from build123d import *

# Parameters (mm, degrees)
PAD_DEPTH       = 17
PAD001_DEPTH    = 2
PAD002_DEPTH    = 1.8
SKETCH003_W     = 32
SKETCH003_H     = 8
PAD003_DEPTH    = 5
SKETCH004_W     = 3.25
SKETCH004_H     = 3.25
POCKET_DEPTH    = 3.1
SKETCH005_W     = 6.497684
SKETCH005_H     = 9.461539
SKETCH005_W_2   = 6.809606
SKETCH005_H_2   = 19.151065
PAD004_DEPTH    = 0.225
CHAMFER_SIZE    = 4
SKETCH006_R     = 0.375
PAD005_DEPTH    = 16
POCKET001_DEPTH = 3
POCKET002_DEPTH = 3
SKETCH009_W     = 42
SKETCH009_H     = 2
PAD006_DEPTH    = 3
CHAMFER001_SIZE = 2


with BuildPart() as part:
    # Sketch → Pad (new body)
    with BuildSketch(Plane.XY):
        with BuildLine():
            Line((-10, 0), (-10, 5))
            Line((-10, 5), (5, 5))
            Line((5, 5), (5, -10))
            Line((5, -10), (0, -10))
            Line((0, -7.05), (0, -10))
            Line((0, -7.05), (0.143534, -7.05))
            ThreePointArc((0.143534, -7.05), (3.05, -6.3), (0.143534, -5.55))
            Line((0, -5.55), (0.143534, -5.55))
            Line((0, 0), (0, -5.55))
            Line((0, 0), (-5.55, 0))
            Line((-5.55, 0), (-5.55, 0.143534))
            ThreePointArc((-5.55, 0.143534), (-6.3, 3.05), (-7.05, 0.143534))
            Line((-7.05, 0), (-7.05, 0.143534))
            Line((-10, 0), (-7.05, 0))
        make_face()
    extrude(amount=-PAD_DEPTH)

    # Sketch001 (on Face16 of Pad) → Pad001 (join)
    with BuildSketch(Plane(origin=(0, 0, -17), x_dir=(1, 0, 0), z_dir=(0, 0, -1))):
        Polygon((5, -5), (-10, -5), (-10, 0), (0, 10), (5, 10), align=None)
    extrude(amount=PAD001_DEPTH)

    # Sketch002 (on Face1 of Pad001) → Pad002 (join)
    with BuildSketch(Plane.XY):
        Polygon((0, -10), (0, 0), (-10, 0), align=None)
    extrude(amount=-PAD002_DEPTH)

    # Sketch003 (on Face10 of Pad002) → Pad003 (join)
    with BuildSketch(Plane.XZ):
        with Locations((-26, -15)):
            Rectangle(SKETCH003_W, SKETCH003_H)
    extrude(amount=-PAD003_DEPTH)

    # Sketch004 (on Face22 of Pad003) → Pocket (cut)
    with BuildSketch(Plane.XZ):
        with Locations((-37.375, -13.375)):
            Rectangle(SKETCH004_W, SKETCH004_H)
    extrude(amount=-POCKET_DEPTH, mode=Mode.SUBTRACT)

    # Sketch005 → Pad004 (join)
    with BuildSketch(Plane(origin=(0, 0, -19), x_dir=(1, 0, 0), z_dir=(0, 0, -1))):
        with Locations((-40.563391, -2.425933)):
            Rectangle(SKETCH005_W, SKETCH005_H)
        with Locations((3.404803, 2.422745)):
            Rectangle(SKETCH005_W_2, SKETCH005_H_2)
    extrude(amount=-PAD004_DEPTH)

    # Chamfer
    chamfer_edges = [part.edges().sort_by_distance(p)[0] for p in [
        (-10, 2.5, -11),
        (5, 5, -9.3875),
    ]]
    chamfer(chamfer_edges, length=CHAMFER_SIZE)

    # Sketch006 (on Face29 of Chamfer) → Pad005 (join)
    with BuildSketch(Plane.XY.offset(-17)):
        with Locations((-6, -3)):
            Circle(SKETCH006_R)
        with Locations((-3, -6)):
            Circle(SKETCH006_R)
    extrude(amount=PAD005_DEPTH)

    # Sketch007 (on Face2 of Pad005) → Pocket001 (cut, symmetric)
    with BuildSketch(Plane.YZ.offset(5)):
        with BuildLine():
            ThreePointArc((-5.25, -5), (-6.25, -4), (-7.25, -5))
            Line((-7.25, -5), (-7.25, -14))
            ThreePointArc((-7.25, -14), (-6.25, -15), (-5.25, -14))
            Line((-5.25, -5), (-5.25, -14))
        make_face()
    extrude(amount=POCKET001_DEPTH, both=True, mode=Mode.SUBTRACT)

    # Sketch008 (on Face5 of Pocket001) → Pocket002 (cut)
    with BuildSketch(Plane(origin=(0, 5, 0), x_dir=(-1, 0, 0), z_dir=(0, 1, 0))):
        with BuildLine():
            ThreePointArc((7.25, -5), (6.25, -4), (5.25, -5))
            Line((5.25, -5), (5.25, -14))
            ThreePointArc((5.25, -14), (6.25, -15), (7.25, -14))
            Line((7.25, -5), (7.25, -14))
        make_face()
    extrude(amount=-POCKET002_DEPTH, mode=Mode.SUBTRACT)

    # Sketch009 (on Face35 of Pocket002) → Pad006 (join)
    with BuildSketch(Plane.XZ):
        with Locations((-21, -18)):
            Rectangle(SKETCH009_W, SKETCH009_H)
    extrude(amount=PAD006_DEPTH)

    # Chamfer001
    chamfer001_edges = [part.edges().sort_by_distance(p)[0] for p in [
        (-42, -3, -18),
    ]]
    chamfer(chamfer001_edges, length=CHAMFER001_SIZE)


solid = part.part
Input: part model. Units: mm. Frame: model coordinates. A direction names the side the tool comes from. Coordinates: 2 decimals unless noted, no trailing zeros. Order: outer loops, then holes, each group sorted by start corner. A loop starts at its lowest first (then second) coordinate and runs counter-clockwise, first axis right, second up.
1. Cut plane D-D, the plane x = 1.5. Return loops of the section in (y, z) (3 decimals), plus the area to 3 significant figures.
Checked values:
outline: (-11.998, -19) - (7.153, -19) - (7.153, -18.775) - (4.5, -18.775) - (4.5, 0) - (-4.75, 0) - (-4.75, -17) - (-7.85, -17) - (-7.85, 0) - (-10, 0) - (-10, -18.775) - (-11.998, -18.775) - close
area: 224 mm2
2. Cut plane C-C, the plane x = -16. Return loops of the section in (y, z), plus the area to 3 significant figures.
Checked values:
outline: (-3, -19) - (5, -19) - (5, -11) - (0, -11) - (0, -17) - (-3, -17) - close
area: 46.0 mm2
3. Access query for faces 4 (the flat face through (-24, -3, -18)), 5 (the cylindrical face through (3.8, -6.3, -15)), 6 (the flat face through (0, -3, -9)). Directions: +Z, -Z, +X, -X, +Y, -Y. A direction counts if a zero-diameter tool reaches every point of the face in a straight line with its end or side. Return the directions, or none.
Checked values:
face 4: +Z, -Z, -X, -Y
face 5: +X
face 6: -Y
4. Cut plane B-B, the plane z = -3.25. Return loops of the section in (x, y) (3 decimals).
Checked values:
outline: (-10, 0) - (-7.05, 0) - (-7.05, 0.144) arc R1.55 cw (long way) to (-5.55, 0.144) - (-5.55, 0) - (0, 0) - (0, -5.55) - (0.144, -5.55) arc R1.55 cw (long way) to (0.144, -7.05) - (0, -7.05) - (0, -10) - (5, -10) - (5, 1) - (1, 5) - (-10, 5) - close; circle Ø0.75 at (-6, -3); circle Ø0.75 at (-3, -6)
5. Cut plane A-A, the plane z = -9.25. Return loops of the section in (x, y) (3 decimals), plus the area to 3 significant figures.
Checked values:
outline: (-12.25, 0) - (-7.05, 0) - (-7.05, 0.144) arc R1.55 cw to (-7.25, 2.725) - (-7.25, 5) - (-12.25, 5) - close; circle Ø0.75 at (-6, -3); (-5.55, 0) - (0, 0) - (0, -5.55) - (0.144, -5.55) arc R1.55 cw to (2.64, -5.25) - (5, -5.25) - (5, 1) - (1, 5) - (-5.25, 5) - (-5.25, 2.64) arc R1.55 cw to (-5.55, 0.144) - close; circle Ø0.75 at (-3, -6); (0, -10) - (5, -10) - (5, -7.25) - (2.725, -7.25) arc R1.55 cw to (0.144, -7.05) - (0, -7.05) - close
area: 106 mm2
6. Draft query along Y for faces 1 (the flat face through (2, -10, -9)), 2 (the flat face through (-1, -1, 0)), 3 (the cylindrical face through (3.8, -6.2, -4)). Return one class per face: +Y half, -Y half, draft (parallel to the pull), parting line (faces both ways), or undercut.
Checked values:
face 1: -Y half
face 2: draft
face 3: undercut
7. Contact query for flat-ended pins moving along their axis: P1, Ø2.5, axis at x = 3.5, z = -10.5, coming from the -Y side; P2, Ø0.6, axis at x = -16, z = -18, coming from the -Y side; P3, Ø6, axis at x = -16, y = -5, coming from the +Z side. Output: stop coordinate, or through.
Checked values:
P1: stops at y = -10
P2: stops at y = -3
P3: stops at z = -17
8. Ray query, line 1 along X through (y, z) = (-3, -11.75) (3 decimals); line 2 along Z through (x, y) = (-1, -2); line 3 along Z through (x, y) = (-30.5, -2). Return the intervals inside material, ascending.
Checked values:
line 1: x = -6.375 to -5.625, 0 to 5
line 2: z = -19 to -17, -1.8 to 0
line 3: z = -19 to -17
